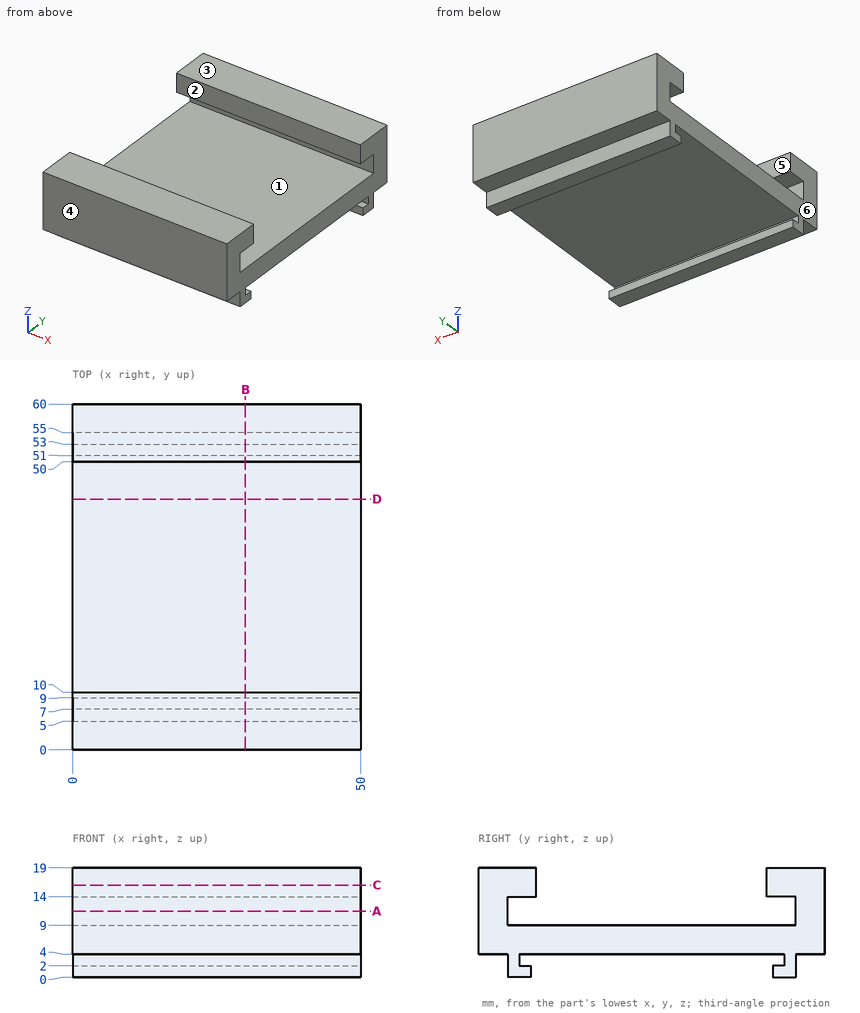
Drawing for the job (mm, zero at the part's lowest x, y, z). A direction names the side the tool comes from. Give positions to 0.01 mm unless a question says otherwise; leave off trailing zeros. Loops run counter-clockwise (first coordinate to the right, second up) from the corner with the lowest first, then second, coordinate; pieces in that order, holes last. Notation, with made-up numbers: M 22.5,78 L 79.5,78 A10 cw 79.5,97 Z; hole C 21,31 d6. An arc over 180 degrees is marked long. Use one line per item in the form item = value.
Item 1: Slice it at A-A (z = 11.5). List the corners of the cut face in (x, y).
Determined:
outline = M 0,0 L 50,0 L 50,5 L 0,5 Z; M 0,55 L 50,55 L 50,60 L 0,60 Z
Item 2: Two-plate mould, pull along Y, no slides. Class the marked faces 4, 5 and 6: pulls with the +Y half, pulls with the -Y half, needs draft (parallel to the pull), parting line crosses it, or undercut.
Determined:
face_4 = pulls with the -Y half
face_5 = undercut
face_6 = needs draft
Item 3: Flat gauge pins, fed straight in: pin 1 (5 mm diameter, centred on y = 41, z = 13.5, fed in from -X); pin 2 (4 mm diameter, centred on y = 37.5, z = 3.5, fed in from +X); pin 3 (0.6 mm diameter, centred on x = 31, z = 1, fed in from +Y); pin 4 (5.5 mm diameter, centred on x = 22, y = 1.5, fed in from -Z). Where does each tip first touch, or does it go through?
Determined:
pin_1 = through
pin_2 = 50
pin_3 = 55
pin_4 = 4
Item 4: Drill centre lines: probe 1 along Z at (x, y) = (41, 8.5); probe 2 along Y at (x, z) = (43.5, 14.5); probe 3 along Y at (x, z) = (14.5, 2.75). Where is each one in solid material? Low to high. Write a range as from..to.
Determined:
probe_1 = 0..2, 4..9, 14..19
probe_2 = 0..10, 50..60
probe_3 = 5..7, 53..55
Item 5: Slice it at B-B (x = 30). List the corners of the cut face in (y, z).
Determined:
outline = M 0,4 L 5,4 L 5,0 L 9,0 L 9,2 L 7,2 L 7,4 L 53,4 L 53,2 L 51,2 L 51,0 L 55,0 L 55,4 L 60,4 L 60,19 L 50,19 L 50,14 L 55,14 L 55,9 L 5,9 L 5,14 L 10,14 L 10,19 L 0,19 Z
Item 6: Which spindle directions (+Z, -Z, +X, -X, +Y, -Y) get a long thin tool onto all of the face, cutting with end or side? Do the marked faces 1, 2 and 3. Say none if no direction does.
Determined:
face_1 = +X, -X
face_2 = +Z, +X, -X
face_3 = +Z, +X, -X, +Y, -Y
Item 7: Slice it at D-D (y = 43.5). List the corners of the cut face in (x, z).
Determined:
outline = M 0,4 L 50,4 L 50,9 L 0,9 Z
Item 8: Slice it at C-C (z = 16). List the corners of the cut face in (x, y).
Determined:
outline = M 0,0 L 50,0 L 50,10 L 0,10 Z; M 0,50 L 50,50 L 50,60 L 0,60 Z
